from build123d import *

# Parameters (mm, degrees)
F0_R     = 390
F0_R_2   = 15
F0_R_3   = 308.25
F1_DEPTH = 42


with BuildPart() as f1:
    # F0 (on Top) → F1 (new body)
    with BuildSketch(Plane.XY):
        Circle(F0_R)
        with Locations((-213.072154, -293.26866)):
            Circle(F0_R_2, mode=Mode.SUBTRACT)
        with Locations((-293.26866, -213.072154)):
            Circle(F0_R_2, mode=Mode.SUBTRACT)
        with Locations((-112.01866, -344.757987)):
            Circle(F0_R_2, mode=Mode.SUBTRACT)
        with Locations((-344.757987, -112.01866)):
            Circle(F0_R_2, mode=Mode.SUBTRACT)
        with Locations((0, -362.5)):
            Circle(F0_R_2, mode=Mode.SUBTRACT)
        with Locations((112.01866, -344.757987)):
            Circle(F0_R_2, mode=Mode.SUBTRACT)
        with Locations((213.072154, -293.26866)):
            Circle(F0_R_2, mode=Mode.SUBTRACT)
        with Locations((293.26866, -213.072154)):
            Circle(F0_R_2, mode=Mode.SUBTRACT)
        with Locations((344.757987, -112.01866)):
            Circle(F0_R_2, mode=Mode.SUBTRACT)
        with Locations((-362.5, 0)):
            Circle(F0_R_2, mode=Mode.SUBTRACT)
        with Locations((-344.757987, 112.01866)):
            Circle(F0_R_2, mode=Mode.SUBTRACT)
        with Locations((-293.26866, 213.072154)):
            Circle(F0_R_2, mode=Mode.SUBTRACT)
        with Locations((-213.072154, 293.26866)):
            Circle(F0_R_2, mode=Mode.SUBTRACT)
        with Locations((-112.01866, 344.757987)):
            Circle(F0_R_2, mode=Mode.SUBTRACT)
        Circle(F0_R_3, mode=Mode.SUBTRACT)
        with Locations((362.5, 0)):
            Circle(F0_R_2, mode=Mode.SUBTRACT)
        with Locations((344.757987, 112.01866)):
            Circle(F0_R_2, mode=Mode.SUBTRACT)
        with Locations((0, 362.5)):
            Circle(F0_R_2, mode=Mode.SUBTRACT)
        with Locations((112.01866, 344.757987)):
            Circle(F0_R_2, mode=Mode.SUBTRACT)
        with Locations((293.26866, 213.072154)):
            Circle(F0_R_2, mode=Mode.SUBTRACT)
        with Locations((213.072154, 293.26866)):
            Circle(F0_R_2, mode=Mode.SUBTRACT)
    extrude(amount=F1_DEPTH)


solid = f1.part
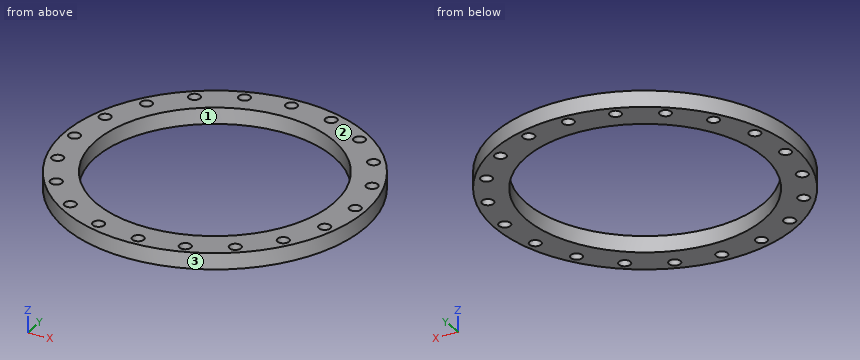
Check sheet for the modelled part. Datum: model origin and axes. Units: mm. Face numbers are marked on the shaded views. Give positions to 0.01 mm unless a question says otherwise; leave off trailing zeros. Loops run counter-clockwise (first coordinate to the right, second up) from the corner with the lowest first, then second, coordinate; pieces in that order, holes last. Notation, with made-up numbers: M 51,70 L 86,70 A26 ccw 86,91 Z; hole C 73,57.5 d6. An arc over 180 degrees is marked long. Return JSON: item names as keys, results as strings. Group by question number.
1. Mould release check, pull along X, two halves, no side actions. Record for the marked faces 1, 2 and 3: released by +X, released by -X, zero draft, split by the parting line, or undercut.
2. Cross-section at A-A on y = 0. Record the boundary of the cut face in (x, z), plus the area to 3 significant figures.
3. Cross-section at D-D on y = 163.5. Record the boundary of the cut face in (x, z), plus the area to 3 significant figures.
4. Cross-section at C-C on z = 13.5. State how many separate pieces and enclosed holes the cut face has, plus the area to 3 significant figures.
5. Thickness scan on L1, parallel to Y at x = 0, z = 31; L2, parallel to Y at x = -346.5, z = 11.5; L3, parallel to Y at x = 123, z = 38.5. Record the ranges inside material, lowest first.
6. Go/stop test with flat-tipped pins: pin 1 (1.5 mm diameter, centred on x = 28, z = 30, fed in from -Y); pin 2 (8 mm diameter, centred on x = -224.5, y = -294.5, fed in from +Z); pin 3 (6 mm diameter, centred on y = 265, z = 31, fed in from +X); pin 4 (8 mm diameter, centred on y = -106, z = 36, fed in from -X). Record where each tip stops, or that it passes through.
Return value:
{
 "1": {"face 1": "undercut", "face 2": "zero draft", "face 3": "split by the parting line"},
 "2": {"outline": "M -390,0 L -377.5,0 L -377.5,42 L -390,42 Z; M -347.5,0 L -308.25,0 L -308.25,42 L -347.5,42 Z; M 308.25,0 L 347.5,0 L 347.5,42 L 308.25,42 Z; M 377.5,0 L 390,0 L 390,42 L 377.5,42 Z", "area": "4,350 mm^2"},
 "3": {"outline": "M -354.07,0 L -261.32,0 L -261.32,42 L -354.07,42 Z; M 261.32,0 L 354.07,0 L 354.07,42 L 261.32,42 Z", "area": "7,790 mm^2"},
 "4": {"separate pieces": "1", "enclosed holes": "21", "area": "165,000 mm^2"},
 "5": {"L1": "-390 to -377.5, -347.5 to -308.25, 308.25 to 347.5, 377.5 to 390", "L2": "-178.99 to -126.92, -97.12 to 97.12, 126.92 to 178.99", "L3": "-370.1 to -354.98, -334.54 to -282.65, 282.65 to 334.54, 354.98 to 370.1"},
 "6": {"pin 1": "y = -389.05", "pin 2": "z = 42", "pin 3": "x = 288.89", "pin 4": "x = -376.43"}
}
